Autodesk Inventor part; units mm, degrees
ref_plane "YZ Plane" through (0, 0, 0) normal (1, 0, 0) x (0, 1, 0)
ref_plane "XZ Plane" through (0, 0, 0) normal (0, 1, 0) x (-1, 0, 0)
ref_plane "XY Plane" through (0, 0, 0) normal (0, 0, 1) x (1, 0, 0)
sketch "Boceto1" plane through (0, 0, 0) normal (0, 1, 0) x (-1, 0, 0)
  line L0 (3.0387, 27.5812) -> (3.0387, -22.4188)
  line L1 (3.0387, -22.4188) -> (11.0387, -22.4188)
  line L2 (11.0387, -22.4188) -> (11.0387, 17.1889)
  line L3 (3.0387, 27.5812) -> (5.0387, 27.5812)
  line L4 (5.0387, 27.5812) -> (11.0387, 17.1889)
  dimension "d0" = 50
  dimension "d1" = 8
  dimension "d3" = 2
  dimension "d69" = 30
extrude "Extrusión1" add sketch "Boceto1" along normal blind 12
sketch "Boceto3" plane through (-11.0387, 0, -22.4188) normal (-1, 0, 0) x (0, 0, 1)
  line L0 (0, 0) -> (0, 12)
  line L1 (39.6077, 0) -> (39.6077, 12)
  line L2 (0, 12) -> (39.6077, 12)
  circle A0 centre (2.5, 6) radius 1.5
  line L3 (9, 3.5) -> (36.5, 3.5)
  line L4 (9, 8.5) -> (36.5, 8.5)
  line L5 (0, 0) -> (39.6077, 0)
  arc A1 (9, 8.5) -> (9, 3.5) centre (9, 6) ccw
  circle A2 centre (9, 6) radius 4.5
  circle A3 centre (36.5, 6) radius 2.5
  dimension "d51" = 3
  dimension "d52" = 2.5
  dimension "d56" = 27.5
  dimension "d63" = 5
  dimension "d64" = 9
  dimension "d65" = 27.5
  dimension "d66" = 9
extrude "Extrusión6" cut sketch "Boceto3" against normal blind 10 contours A0 | A1 L4 A2 L3 | A2 L4 A3 L3 | A3 picked at (10.5, 6)
thread "Thread1"
properties part number "Chaponete" material "Steel, High Strength, Low Alloy"
Check sheet for the modelled part. Datum: model origin and axes. Units: mm. A direction names the side the tool comes from. Give positions to 0.01 mm unless a question says otherwise; leave off trailing zeros. Loops run counter-clockwise (first coordinate to the right, second up) from the corner with the lowest first, then second, coordinate; pieces in that order, holes last. Notation, with made-up numbers: M -18.75,-11.5 L 17.25,-11.5 A31 ccw 17.25,26.5 Z; hole C -40,71 d6. An arc over 180 degrees is marked long. Return JSON: item names as keys, results as strings. Group by question number.
1. Cross-section at D-D on y = 1. Record the boundary of the cut face in (x, z), plus the area to 3 significant figures.
2. Cross-section at A-A on y = 6. Record the boundary of the cut face in (x, z), plus the area to 3 significant figures.
3. Mould release check, pull along Y, two halves, no side actions. Record for faces 3 (the flat face through (-7, 8.5, 0)), 4 (the flat face through (-4, 6, 27.581)), 5 (the cylindrical face through (-7.09, 5.95, 16.58)), 6 (the flat face through (-7, 0, 3)): released by +Y, released by -Y, zero draft, split by the parting line, or undercut.
4. Cross-section at B-B on z = 11. Record the boundary of the cut face in (x, y).
5. Thickness scan on L1, parallel to Y at x = -7.75, z = 0; L2, parallel to Z at x = -6.25, y = 6.5; L3, parallel to Y at x = -6.75, z = 15. Record the ranges inside material, lowest first.
6. Tool access check on faces 1 (the cylindrical face through (-7.09, 6.05, -15.92)), 2 (the flat face through (-7.997, 5.916, 22.458)). Record the directions out of +Z, -Z, +X, -X, +Y, -Y that give a thin tool (end or side, any length) a straight path to the whole face; none if there is none.
7. Go/stop test with flat-tipped pins: pin 1 (1.5 mm diameter, centred on x = -9, y = 4.5, fed in from +Z); pin 2 (2 mm diameter, centred on x = -8.5, y = 7, fed in from +Z); pin 3 (3 mm diameter, centred on y = 6.5, z = 1.5, fed in from +X). Record where each tip stops, or that it passes through.
8. Cross-section at C-C on x = -4.5. Record the boundary of the cut face in (y, z), plus the area to 3 significant figures.
Return value:
{
 "1": {"outline": "M -11.04,-22.42 L -3.04,-22.42 L -3.04,27.58 L -5.04,27.58 L -11.04,17.19 Z", "area": "369 mm^2"},
 "2": {"outline": "M -11.04,-22.42 L -3.04,-22.42 L -3.04,-21.42 L -11.04,-21.42 Z; M -11.04,-18.42 L -3.04,-18.42 L -3.04,-15.92 L -11.04,-15.92 Z; M -11.04,16.58 L -3.04,16.58 L -3.04,27.58 L -5.04,27.58 L -11.04,17.19 Z", "area": "84.8 mm^2"},
 "3": {"face 3": "undercut", "face 4": "zero draft", "face 5": "undercut", "face 6": "released by -Y"},
 "4": {"outline": "M -11.04,0 L -3.04,0 L -3.04,3.5 L -11.04,3.5 Z; M -11.04,8.5 L -3.04,8.5 L -3.04,12 L -11.04,12 Z"},
 "5": {"L1": "0 to 3.5, 8.5 to 12", "L2": "-22.42 to -21.33, -18.5 to -15.87, 16.53 to 25.48", "L3": "0 to 3.67, 8.33 to 12"},
 "6": {"face 1": "+X, -X", "face 2": "+Z, -X, +Y, -Y"},
 "7": {"pin 1": "z = 22.02", "pin 2": "z = 23.32", "pin 3": "through"},
 "8": {"outline": "M 0,-22.42 L 12,-22.42 L 12,27.58 L 0,27.58 Z; hole M 3.5,-13.42 A2.5 ccw 8.5,-13.42 L 8.5,14.08 A2.5 ccw 3.5,14.08 Z; hole C 6,-19.92 d3", "area": "436 mm^2"}
}
